Check sheet for the modelled part. Datum: model origin and axes. Units: mm. Face numbers are marked on the shaded views. A direction names the side the tool comes from. Coordinates: 2 decimals unless noted, no trailing zeros. Loops run counter-clockwise (first coordinate to the right, second up) from the corner with the lowest first, then second, coordinate; pieces in that order, holes last. Notation, with made-up numbers: (47.25, -1.5) - (81.25, -1.5) arc R31 cw to (81.25, 35.5) - close; hole circle Ø6 at (24.5, 58.25). An arc over 180 degrees is marked (long way). Write each question's results on one line, items separated by ' | '. Start each with the question number.
1. Cross-section at A-A (x = 30). Record the cut outline in (y, z).
2. Cross-section at D-D (y = 21). Record the cut outline in (x, z), and give its area (3 significant figures).
3. Gauge pin test, flat ends, axial feed: P1, Ø4, axis at x = 9, y = 66.5, coming from the -Z side; P2, Ø1.5, axis at y = 66.5, z = -12, coming from the +X side; P3, Ø7, axis at x = 9, z = -17.5, coming from the +Y side. Record the tip position at first contact, or that the pin passes through.
4. Draft check along Y on the marked faces 6, 7 and 8. Enter one of: released by +Y, released by -Y, zero draft, split by the parting line, or undercut.
5. Cross-section at C-C (y = 10). Record the cut outline in (x, z).
6. Thickness scan on line 1 (X direction, y = 3.5, z = 0); line 2 (X direction, y = 1.95, z = 0); line 3 (Z direction, x = 6, y = 65). Record the ranges inside material, lowest first. Write a range as [from, to].
7. Tool access check on the marked faces 1, 2, 3, 4 and 5. Record the directions out of +Z, -Z, +X, -X, +Y, -Y that give a thin tool (end or side, any length) a straight path to the whole face; none if there is none.
8. Cross-section at B-B (y = 35). Record the cut outline in (x, z), and give its area (3 significant figures).
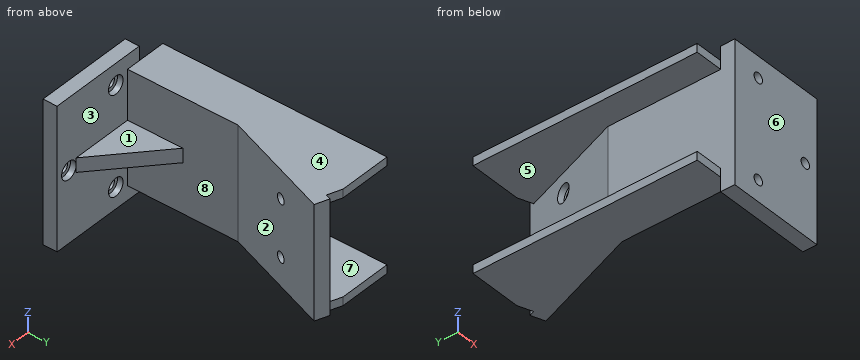
```python
from build123d import *

# Parameters (mm, degrees)
SKETCH_2_W          = 5
SKETCH_2_H          = 40
CUT_EXTRUDE_1_REACH = 90.301
SKETCH_3_R          = 1.8
SKETCH_6_W          = 30
SKETCH_6_H          = 40
EXTRUDE_1_DEPTH     = 5
CUT_EXTRUDE_2_REACH = 95.593
SKETCH_8_R          = 1.8
SKETCH_9_W          = 35
SKETCH_9_H          = 5
EXTRUDE_2_DEPTH     = 5
SKETCH_10_R         = 3.1
CUT_EXTRUDE_3_DEPTH = 2
SKETCH_11_R         = 3.1
CUT_EXTRUDE_4_DEPTH = 2
EXTRUDE_4_DEPTH     = 3
RIB_5_REACH         = 96.788
SKETCH_21_WALL_W    = 220.937961122
SKETCH_21_WALL_H    = 5


with BuildPart() as part:
    # 扫描1: sweep along a path in 草图1
    with BuildLine(Plane.XY) as sweep_1_path:
        Line((0, 0), (0, 45))
        Line((0, 45), (14.36484602, 84.467090073))
    # 草图2 → 扫描1 (sweep)
    with BuildSketch(Plane(origin=(0, 0, 0), x_dir=(1, 0, 0), z_dir=(0, 1, 0))):
        with Locations((2.5, 0)):
            Rectangle(SKETCH_2_W, SKETCH_2_H)
    sweep(path=sweep_1_path.line, transition=Transition.RIGHT)

    # 草图3 → 切除-拉伸1 (cut, up to next)
    with BuildSketch(Plane(origin=(-14.462721218, 5.26400003, 0), x_dir=(0, 0, 1), z_dir=(-0.9396926207859081, 0.3420201433256695, 0)), mode=Mode.PRIVATE) as cut_extrude_1_sk1:
        with Locations(Location((-10, 66.286167935, 0), (0, 0, 270))):
            Circle(SKETCH_3_R)
    cut_extrude_1_tool1 = extrude(cut_extrude_1_sk1.sketch, amount=-CUT_EXTRUDE_1_REACH, mode=Mode.PRIVATE) & part.part
    # 草图3 → 切除-拉伸1 (cut, up to next)
    with BuildSketch(Plane(origin=(-14.462721218, 5.26400003, 0), x_dir=(0, 0, 1), z_dir=(-0.9396926207859081, 0.3420201433256695, 0)), mode=Mode.PRIVATE) as cut_extrude_1_sk2:
        with Locations(Location((10, 66.286167935, 0), (0, 0, 270))):
            Circle(SKETCH_3_R)
    cut_extrude_1_tool2 = extrude(cut_extrude_1_sk2.sketch, amount=-CUT_EXTRUDE_1_REACH, mode=Mode.PRIVATE) & part.part
    add(cut_extrude_1_tool1.solids().sort_by_distance((8.208483, 67.552623, -10))[0], mode=Mode.SUBTRACT)
    add(cut_extrude_1_tool2.solids().sort_by_distance((8.208483, 67.552623, 10))[0], mode=Mode.SUBTRACT)

    # 草图6 → 凸台-拉伸1 (add)
    with BuildSketch(Plane.XZ):
        with Locations((20, 0)):
            Rectangle(SKETCH_6_W, SKETCH_6_H)
    extrude(amount=-EXTRUDE_1_DEPTH)

    # 草图8 → 切除-拉伸2 (cut, up to next)
    with BuildSketch(Plane.XZ, mode=Mode.PRIVATE) as cut_extrude_2_sk1:
        with Locations(Location((10, 17.5, 0), (0, 0, 270))):
            Circle(SKETCH_8_R)
    cut_extrude_2_tool1 = extrude(cut_extrude_2_sk1.sketch, amount=-CUT_EXTRUDE_2_REACH, mode=Mode.PRIVATE) & part.part
    # 草图8 → 切除-拉伸2 (cut, up to next)
    with BuildSketch(Plane.XZ, mode=Mode.PRIVATE) as cut_extrude_2_sk2:
        with Locations(Location((10, -17.5, 0), (0, 0, 270))):
            Circle(SKETCH_8_R)
    cut_extrude_2_tool2 = extrude(cut_extrude_2_sk2.sketch, amount=-CUT_EXTRUDE_2_REACH, mode=Mode.PRIVATE) & part.part
    # 草图8 → 切除-拉伸2 (cut, up to next)
    with BuildSketch(Plane.XZ, mode=Mode.PRIVATE) as cut_extrude_2_sk3:
        with Locations(Location((30, 0, 0), (0, 0, 270))):
            Circle(SKETCH_8_R)
    cut_extrude_2_tool3 = extrude(cut_extrude_2_sk3.sketch, amount=-CUT_EXTRUDE_2_REACH, mode=Mode.PRIVATE) & part.part
    add(cut_extrude_2_tool1.solids().sort_by_distance((10, 0, 17.5))[0], mode=Mode.SUBTRACT)
    add(cut_extrude_2_tool2.solids().sort_by_distance((10, 0, -17.5))[0], mode=Mode.SUBTRACT)
    add(cut_extrude_2_tool3.solids().sort_by_distance((30, 0, 0))[0], mode=Mode.SUBTRACT)

    # 草图9 → 凸台-拉伸2 (add)
    with BuildSketch(Plane.XZ):
        with Locations((17.5, 22.5)):
            Rectangle(SKETCH_9_W, SKETCH_9_H)
        with Locations((17.5, -22.5)):
            Rectangle(SKETCH_9_W, SKETCH_9_H)
    extrude(amount=-EXTRUDE_2_DEPTH)

    # 草图10 → 切除-拉伸3 (cut)
    with BuildSketch(Plane(origin=(0, 5, 0), x_dir=(1, 0, 0), z_dir=(0, 1, 0))):
        with Locations(Location((10, -17.5, 0), (0, 0, 270))):
            Circle(SKETCH_10_R)
        with Locations(Location((10, 17.5, 0), (0, 0, 270))):
            Circle(SKETCH_10_R)
        with Locations(Location((30, 0, 0), (0, 0, 270))):
            Circle(SKETCH_10_R)
    extrude(amount=-CUT_EXTRUDE_3_DEPTH, mode=Mode.SUBTRACT)

    # 草图11 → 切除-拉伸4 (cut)
    with BuildSketch(Plane(origin=(-14.462721218, 5.26400003, 0), x_dir=(0, 0, 1), z_dir=(-0.9396926207859081, 0.3420201433256695, 0))):
        with Locations(Location((-10, 66.286167935, 0), (0, 0, 270))):
            Circle(SKETCH_11_R)
        with Locations(Location((10, 66.286167935, 0), (0, 0, 270))):
            Circle(SKETCH_11_R)
    extrude(amount=-CUT_EXTRUDE_4_DEPTH, mode=Mode.SUBTRACT)

    # 草图15 → 凸台-拉伸4 (add)
    with BuildSketch(Plane(origin=(0, 0, -20), x_dir=(-1, 0, 0), z_dir=(0, 0, -1))):
        Polygon((-8.680805733, 84.407556003), (-13.680805733, 82.587704831), (0, 45), (0, 5), (10, 5), (10, 84.407556003), align=None)
    extrude_4 = extrude(amount=-EXTRUDE_4_DEPTH)

    # 镜向2: 凸台-拉伸4 across plane
    add(extrude_4.mirror(Plane(origin=(0, 0, 0), x_dir=(1, 0, 0), z_dir=(0, 0, -1))))

    # 草图21 wall → 筋5 (add, up to next)
    with BuildSketch(Plane(origin=(15.95, 14.779591274, 0), x_dir=(0.745842716131, -0.666122093009, 0), z_dir=(-0.666122093009, -0.745842716131, 0)), mode=Mode.PRIVATE) as rib_5_sk1:
        Rectangle(SKETCH_21_WALL_W, SKETCH_21_WALL_H)
    rib_5_tool1 = extrude(rib_5_sk1.sketch, amount=RIB_5_REACH, mode=Mode.PRIVATE) - part.part
    add(rib_5_tool1.solids().sort_by_distance((15.95, 14.779591274, 0))[0])


solid = part.part
```
Established:
1) outline: (0, -25) - (5, -25) - (5, -3.1) - (3, -3.1) - (3, -1.8) - (0, -1.8) - close; (0, 1.8) - (3, 1.8) - (3, 3.1) - (5, 3.1) - (5, 25) - (0, 25) - close
2) outline: (-10, -20) - (5, -20) - (5, -2.5) - (8.99, -2.5) - (8.99, 2.5) - (5, 2.5) - (5, 20) - (-10, 20) - (-10, 17) - (0, 17) - (0, -17) - (-10, -17) - close | area: 280 mm^2
3) P1: z = -20 | P2: x = 13.42 | P3: y = 84.41
4) face 6: released by -Y | face 7: zero draft | face 8: undercut
5) outline: (-10, -20) - (5, -20) - (5, -2.5) - (21.3, -2.5) - (21.3, 2.5) - (5, 2.5) - (5, 20) - (-10, 20) - (-10, 17) - (0, 17) - (0, -17) - (-10, -17) - close
6) line 1: [0, 26.9], [33.1, 35] | line 2: [0, 28.2], [31.8, 35] | line 3: [-20, -17], [17, 20]
7) face 1: +Z, +X | face 2: +Z, -Z, +X | face 3: +X | face 4: +Z, +X, -X, +Y | face 5: -X, +Y
8) outline: (-10, -20) - (5, -20) - (5, 20) - (-10, 20) - (-10, 17) - (0, 17) - (0, -17) - (-10, -17) - close | area: 260 mm^2
